The model under review builds one solid part; all positions refer to its coordinate system, in mm. A direction names the side the tool comes from. Give positions to 0.01 mm unless a question says otherwise; leave off trailing zeros. Order: outer loops, then holes, each group sorted by start corner. A loop starts at its lowest first (then second) coordinate and runs counter-clockwise, first axis right, second up. Notation, with made-up numbers: (77.5, -33.75) - (100.5, -33.75) arc R26 cw to (100.5, 0.25) - close; hole circle Ø10 at (-29.75, -15). An arc over 180 degrees is marked (long way). Use CSV: the item, a comma, the result in double quotes. Start each with the question number.
1. Take a section at B-B, the plane y = 0. State the section outline as (x, z) points, then the cut area to 3 significant figures.
2. Take a section at C-C, the plane x = 15. State the section outline as (y, z) points, then the cut area to 3 significant figures.
3. Take a section at A-A, the plane x = 25.5. State the section outline as (y, z) points.
4. To check wall thickness, follow line 1 (Z direction, x = 4, y = -20); line 2 (Y direction, x = 15, z = -29); line 3 (X direction, y = 1, z = -17). State the ranges of each line that lie inside material, in increasing order. Write a range as [from, to].
5. Take a section at D-D, the plane y = 16.5. State the section outline as (x, z) points.
6. Draft analysis for pull direction Y (two halves, no side actions). For faces 1 (the flat face through (21, -6, -25)), 2 (the cylindrical face through (21.349, -4.868, 29.93)), 3 (the cylindrical face through (21.349, -4.868, -30.07)), 4 (the flat face through (41, -25, 0)), state which applies: released by +Y, released by -Y, zero draft, split by the parting line, or undercut.
7. Machinability: for faces 5 (the flat face through (25, 0, 35)), 6 (the cylindrical face through (39, 0, 23)), which of the approach directions +Z, -Z, +X, -X, +Y, -Y give a long, thin tool a straight path to every point of the face, cutting with its end or side? Answer none if there is none.
```python
from build123d import *

# Parameters (mm, degrees)
F1_DEPTH = 25
F4_D     = 16
F5_R     = 5


with BuildPart() as f1:
    # F0 (on Front) → F1 (new body, symmetric)
    with BuildSketch(Plane.XZ):
        Polygon((40, 0), (50, 0), (50, 35), (0, 35), (0, 25), (40, 25), align=None)
    extrude(amount=F1_DEPTH, both=True)

    # F2: F1 across plane


with BuildPart() as f1_1:
    add(f1.part)
    add(f1.part.mirror(Plane.XY))

    # F4 (through all)
    with Locations(Plane.XY.offset(35)):
        with Locations((15, 0)):
            Hole(F4_D / 2)

    # F5
    f5_edges = [f1_1.edges().sort_by_distance(p)[0] for p in [
        (40, 0, 25),
        (40, 0, -25),
    ]]
    fillet(f5_edges, radius=F5_R)


solid = f1_1.part
```
Determined:
1,outline,"(0, -35) - (7, -35) - (7, -25) - (0, -25) - close; (0, 25) - (7, 25) - (7, 35) - (0, 35) - close; (23, -35) - (50, -35) - (50, 35) - (23, 35) - (23, 25) - (35, 25) arc R5 cw to (40, 20) - (40, -20) arc R5 cw to (35, -25) - (23, -25) - close"
1,area,"1,190 mm²"
2,outline,"(-25, -35) - (-8, -35) - (-8, -25) - (-25, -25) - close; (-25, 25) - (-8, 25) - (-8, 35) - (-25, 35) - close; (8, -35) - (25, -35) - (25, -25) - (8, -25) - close; (8, 25) - (25, 25) - (25, 35) - (8, 35) - close"
2,area,"680 mm²"
3,outline,"(-25, -35) - (25, -35) - (25, -25) - (-25, -25) - close; (-25, 25) - (25, 25) - (25, 35) - (-25, 35) - close"
4,line 1,"z = [-35, -25], [25, 35]"
4,line 2,"y = [-25, -8], [8, 25]"
4,line 3,"x = [40, 50]"
5,outline,"(0, -35) - (50, -35) - (50, 35) - (0, 35) - (0, 25) - (35, 25) arc R5 cw to (40, 20) - (40, -20) arc R5 cw to (35, -25) - (0, -25) - close"
6,face 1,"zero draft"
6,face 2,"undercut"
6,face 3,"undercut"
6,face 4,"released by -Y"
7,face 5,"+Z, +X, -X, +Y, -Y"
7,face 6,"-X, +Y, -Y"
